Read the model definition and answer for the solid it produces. Units are mm, in the model's axes. Face numbers are marked on the shaded views. A direction names the side the tool comes from. Coordinates: 2 decimals unless noted, no trailing zeros. Order: outer loops, then holes, each group sorted by start corner. A loop starts at its lowest first (then second) coordinate and runs counter-clockwise, first axis right, second up.
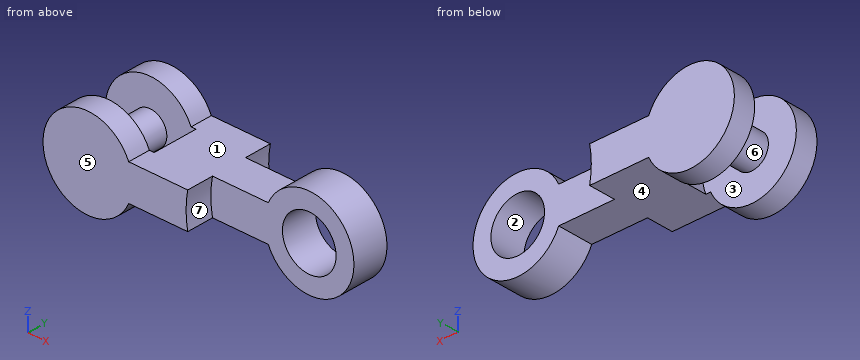
```python
from build123d import *

# Parameters (mm, degrees)
SKETCH2_R               = 5
SKETCH2_R_2             = 1.875
SKETCH2_R_3             = 3
BOSS_EXTRUDE1_DEPTH     = 5
CUT_EXTRUDE1_START      = 2
SKETCH3_R               = 11
CUT_EXTRUDE1_DEPTH      = 4
SKETCH3_3_R             = 5.5
CUT_EXTRUDE2_DEPTH      = 2.55
CUT_EXTRUDE2_DEPTH_BACK = 2.5
SKETCH5_R               = 1.875
BOSS_EXTRUDE2_DEPTH     = 10


with BuildPart() as part:
    # Sketch2 → Boss-Extrude1 (new body, symmetric)
    with BuildSketch(Plane(origin=(0, 0, 0), x_dir=(1, 0, 0), z_dir=(0, 1, 0))):
        with Locations((-11, 0)):
            Circle(SKETCH2_R)
        with Locations((-11, 0)):
            Circle(SKETCH2_R_2, mode=Mode.SUBTRACT)
        with Locations((11, 0)):
            Circle(SKETCH2_R)
        with Locations((11, 0)):
            Circle(SKETCH2_R_3, mode=Mode.SUBTRACT)
        with BuildLine():
            ThreePointArc((-6, 0), (-6.105468435, -1.021548218), (-6.417424305, -2))
            Line((-6.417424305, -2), (6.417424305, -2))
            ThreePointArc((6.417424305, -2), (6, 0), (6.417424305, 2))
            Line((6.417424305, 2), (-6.417424305, 2))
            ThreePointArc((-6.417424305, 2), (-6.105468435, 1.021548218), (-6, 0))
        make_face()
    extrude(amount=BOSS_EXTRUDE1_DEPTH, both=True)

    # Sketch3 → Cut-Extrude1 (cut, through all)
    with BuildSketch(Plane(origin=(0, 0, 0), x_dir=(1, 0, 0), z_dir=(0, 1, 0)).offset(CUT_EXTRUDE1_START)):
        with Locations((11, 0)):
            Circle(SKETCH3_R)
    cut_extrude1 = extrude(amount=CUT_EXTRUDE1_DEPTH, mode=Mode.SUBTRACT)

    # Mirror2: Cut-Extrude1 across plane
    add(cut_extrude1.mirror(Plane.ZX), mode=Mode.SUBTRACT)

    # Sketch3<3> → Cut-Extrude2 (cut, two sides)
    with BuildSketch(Plane(origin=(0, 0, 0), x_dir=(1, 0, 0), z_dir=(0, 1, 0))) as cut_extrude2_sk:
        with Locations((-11, 0)):
            Circle(SKETCH3_3_R)
    extrude(amount=CUT_EXTRUDE2_DEPTH, mode=Mode.SUBTRACT)
    extrude(cut_extrude2_sk.sketch, amount=-CUT_EXTRUDE2_DEPTH_BACK, mode=Mode.SUBTRACT)

    # Sketch5 → Boss-Extrude2 (add)
    with BuildSketch(Plane(origin=(0, 5, 0), x_dir=(1, 0, 0), z_dir=(0, 1, 0))):
        with Locations((-11, 0)):
            Circle(SKETCH5_R)
    extrude(amount=-BOSS_EXTRUDE2_DEPTH)


solid = part.part
```
1) A cutting plane is placed at B-B, the plane x = 11. Determine the outline of the cut face in (y, z), and give its area (3 significant figures).
A:
outline: (-2, -5) - (2, -5) - (2, -3) - (-2, -3) - close; (-2, 3) - (2, 3) - (2, 5) - (-2, 5) - close
area: 16.0 mm2
2) A cutting plane is placed at C-C, the plane y = -1.5. Determine the outline of the cut face in (x, z) (3 decimals).
A:
outline: circle Ø3.75 at (-11, 0); (-5.877, -2) - (6.417, -2) arc R5 ccw (long way) to (6.417, 2) - (-5.877, 2) arc R5.5 cw to start; hole circle Ø6 at (11, 0)
3) Which of the six approach directions +Z, -Z, +X, -X, +Y, -Y give full straight-line access (tool end or side, diameter ignored) to the marked faces 1, 2 and 3?
A:
face 1: +Z, +Y, -Y
face 2: +Y, -Y
face 3: none
4) Determine the mould class of the marked faces 4, 5, 6 and 7 for opening direction Z: pulls with the +Z half, pulls with the -Z half, needs draft (parallel to the pull), parting line crosses it, or undercut.
A:
face 4: pulls with the -Z half
face 5: needs draft
face 6: parting line crosses it
face 7: undercut
5) Flat-ended cylindrical pins translate along their axes: pin 1 Ø1 at (x, z) = (6, -0.5) entering from -Y; pin 2 Ø4 at (y, z) = (2.5, 2.5) entering from +X; pin 3 Ø1.5 at (x, y) = (3, -3) entering from -Z; pin 4 Ø5 at (x, z) = (11, 1.5) entering from +Y. Find the tip coordinate at first contact, or state that the pin passes through.
A:
pin 1: stops at y = -2
pin 2: stops at x = 15.97
pin 3: passes through
pin 4: stops at y = 2
6) A cutting plane is placed at D-D, the plane z = -3.5. Determine the outline of the cut face in (x, y), and give its area (3 significant figures).
A:
outline: (-14.57, -5) - (-7.43, -5) - (-7.43, -2.5) - (-14.57, -2.5) - close; (-14.57, 2.55) - (-7.43, 2.55) - (-7.43, 5) - (-14.57, 5) - close; (7.43, -2) - (14.57, -2) - (14.57, 2) - (7.43, 2) - close
area: 63.9 mm2
7) Straight lines are drawn through the part: line 1 (Z direction, x = 11, y = -0.2); line 2 (Y direction, x = -9.5, z = 2.75); line 3 (Y direction, x = 9, z = 4.5). For each, find the intervals that lie inside material, in ascending order.
A:
line 1: z = -5 to -3, 3 to 5
line 2: y = -5 to -2.5, 2.55 to 5
line 3: y = -2 to 2
8) A cutting plane is placed at A-A, the plane z = 0. Determine the outline of the cut face in (x, y) (3 decimals).
A:
outline: (-16, -5) - (0, -5) - (0, -2) - (8, -2) - (8, 2) - (0, 2) - (0, 5) - (-16, 5) - (-16, 2.55) - (-12.875, 2.55) - (-12.875, -2.5) - (-16, -2.5) - close; (14, -2) - (16, -2) - (16, 2) - (14, 2) - close; hole (-9.125, -2.5) - (-5.5, -2.5) - (-5.5, 2.55) - (-9.125, 2.55) - close
